Source: CAD feature listing. Evaluate the final solid. Frame: model axes, mm. Face numbers are marked on the shaded views. A direction names the side the tool comes from. Give positions to 0.01 mm unless a question says otherwise; leave off trailing zeros. Loops run counter-clockwise (first coordinate to the right, second up) from the corner with the lowest first, then second, coordinate; pieces in that order, holes last. Notation, with made-up numbers: (-31, 23) -> (19, 23) arc R34 ccw to (19, 62) -> close; hole circle Ø2 at (-24.5, 7.5). An arc over 180 degrees is marked (long way). Return JSON: item names as keys, results as strings. Group by question number.
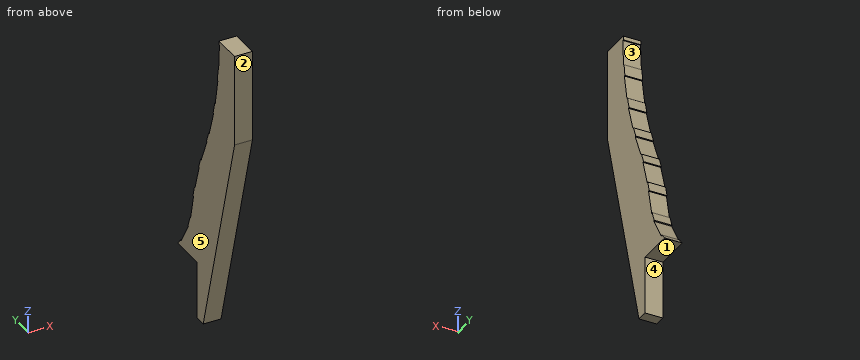
```python
from build123d import *

# Parameters (mm, degrees)
F1_DEPTH = 44
F3_DEPTH = 44.001


with BuildPart() as f1:
    # F0 (on Right) → F1 (new body)
    with BuildSketch(Plane.YZ):
        with BuildLine():
            Line((0, -143), (0, 0))
            Line((0, 0), (89.5, 0))
            Line((89.5, 0), (89.5, 0.135534))
            ThreePointArc((89.5, 0.135534), (48.246456, 57.869699), (25.678122, 125.143461))
            ThreePointArc((25.678122, 125.143461), (2.97396, 218.234418), (-31.413874, 307.670888))
            ThreePointArc((-31.413874, 307.670888), (-82.652853, 460.62607), (-100, 621))
            Line((-100, 621), (-172, 621))
            Line((-172, 621), (-172, 394.415316))
            Line((-172, 394.415316), (-28, -143))
            Line((-28, -143), (0, -143))
        make_face()
    extrude(amount=-F1_DEPTH)

    # F2 (on face) → F3 (cut, through all)
    with BuildSketch(Plane.YZ):
        Polygon((74.071089, 13.776057), (76.205662, 15.077441), (41.849131, 71.430158), (39.714558, 70.128774), align=None)
        Polygon((30.361442, 95.267272), (32.802788, 95.805631), (19.715373, 160.494236), (18.590111, 160.257162), (16.148766, 159.718803), align=None)
        Polygon((10.012695, 184.7665), (12.399741, 185.509475), (-3.192727, 249.82656), (-7.214805, 248.527485), (-9.601851, 247.78451), align=None)
        Polygon((-18.74354, 271.839235), (-16.449247, 272.832322), (-40.185015, 334.475862), (-42.666724, 333.401653), (-44.961017, 332.408567), align=None)
        Polygon((-55.647484, 359.630059), (-53.267308, 360.394756), (-73.455309, 423.231407), (-75.835485, 422.46671), align=None)
        Polygon((-92.64633, 516.231548), (-95.104054, 515.773736), (-83.017833, 450.889815), (-80.560108, 451.347626), align=None)
        Polygon((-98.662946, 545.231548), (-96.162946, 545.231548), (-99.936382, 611.231548), (-102.436382, 611.231548), align=None)
    extrude(amount=-F3_DEPTH, mode=Mode.SUBTRACT)


solid = f1.part
```
1) Material intervals for line 1 (Z direction, x = -29, y = 76); line 2 (Y direction, x = -20.5, z = 186); line 3 (Y direction, x = -27.5, z = 539.5), sorted ascending.
2) Cut plane A-A on y = -62.5. Return loops of the section in (x, z), then the cut area to 3 significant figures.
3) Mould query, pull axis Z, two halves, no side actions, for the marked faces 1, 2 and 3. Classes: released by +Z, released by -Z, zero draft, split by the parting line, or undercut.
4) Cut plane B-B on z = -23. Return loops of the section in (x, y), then the cut area to 3 significant figures.
5) Reachability of the marked faces 4 and 5 from +Z, -Z, +X, -X, +Y, -Y: full face, straight path, thin tool, end or side. Return the list, or none.
6) Contact query for flat-ended pins moving along their axis: P1, Ø1, axis at x = -22, z = -35, coming from the -Y side; P2, Ø13, axis at x = -14, z = -72, coming from the +Y side; P3, Ø8, axis at x = -10, z = 513.5, coming from the +Y side. Output: stop coordinate, or through.
Calculated:
{
 "1": {"line 1": "0 to 14.95", "line 2": "-116.16 to 9.63", "line 3": "-172 to -95.56"},
 "2": {"outline": "(-44, -14.24) -> (0, -14.24) -> (0, 380.96) -> (-44, 380.96) -> close", "area": "17,400 mm2"},
 "3": {"face 1": "released by -Z", "face 2": "zero draft", "face 3": "undercut"},
 "4": {"outline": "(-44, -60.15) -> (0, -60.15) -> (0, 0) -> (-44, 0) -> close", "area": "2,650 mm2"},
 "5": {"face 4": "-Z, +X, -X, +Y", "face 5": "+Z, -Z, -X, +Y, -Y"},
 "6": {"P1": "y = -57.07", "P2": "y = 0", "P3": "y = -92.65"}
}
